The figure shows three views and two pictorial views of one solid part (mm, origin at its lowest corner). Answer the questions. Coordinates: 2 decimals unless noted, no trailing zeros. Loops run counter-clockwise (first coordinate to the right, second up) from the corner with the lowest first, then second, coordinate; pieces in that order, holes last. Notation, with made-up numbers: (30.5, -9) -> (43.5, -9) arc R8 cw to (43.5, 6) -> close; hole circle Ø10 at (89.25, -9). An arc over 180 degrees is marked (long way). Answer in a Markdown table with one row per item.
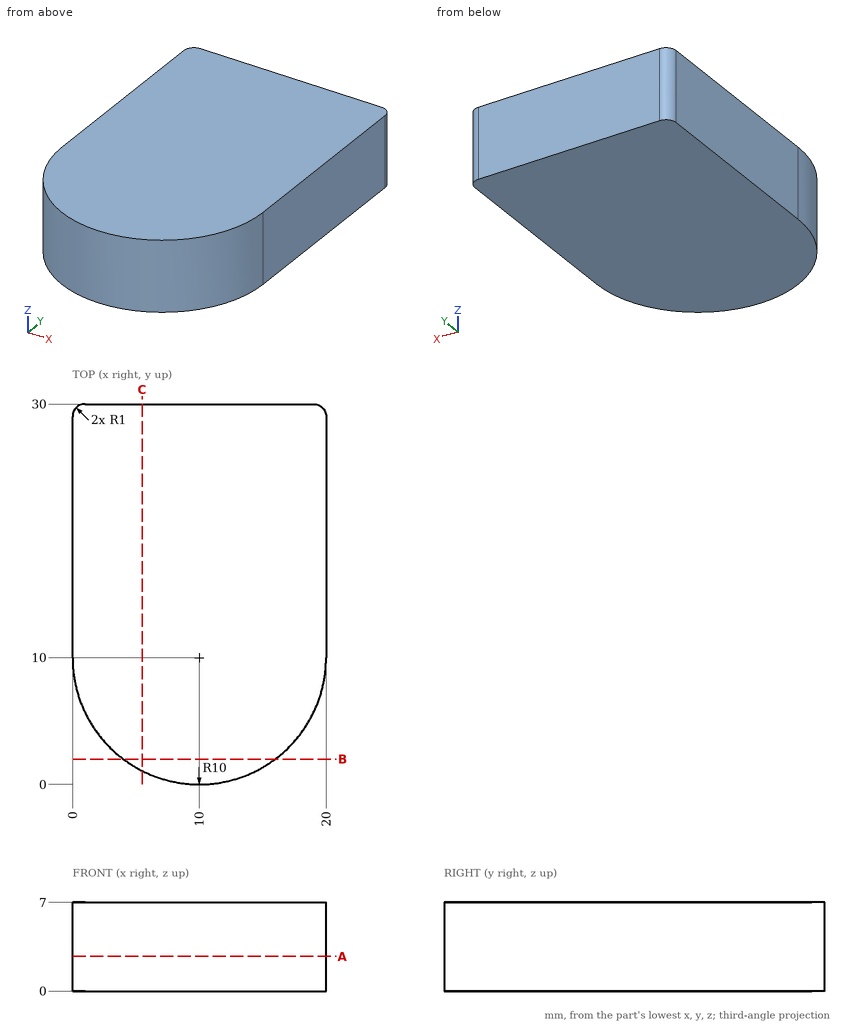
Item 1: A cutting plane is placed at B-B, the plane y = 2. Determine the outline of the cut face in (x, z), plus the area to 3 significant figures.
Findings below:
| item | result |
|---|---|
| outline | (4, 0) -> (16, 0) -> (16, 7) -> (4, 7) -> close |
| area | 84.0 mm2 |
Item 2: A cutting plane is placed at A-A, the plane z = 2.75. Determine the outline of the cut face in (x, y), plus the area to 3 significant figures.
Findings below:
| item | result |
|---|---|
| outline | (0, 10) arc R10 ccw to (20, 10) -> (20, 29) arc R1 ccw to (19, 30) -> (1, 30) arc R1 ccw to (0, 29) -> close |
| area | 557 mm2 |
Item 3: Flat-ended cylindrical pins translate along their axes: pin 1 Ø1.5 at (x, y) = (10.5, 3.5) entering from -Z; pin 2 Ø1 at (x, z) = (5, 3.5) entering from -Y. Find the tip coordinate at first contact, or state that the pin passes through.
Findings below:
| item | result |
|---|---|
| pin 1 | stops at z = 0 |
| pin 2 | stops at y = 1.07 |
Item 4: A cutting plane is placed at C-C, the plane x = 5.5. Determine the outline of the cut face in (y, z), plus the area to 3 significant figures.
Findings below:
| item | result |
|---|---|
| outline | (1.07, 0) -> (30, 0) -> (30, 7) -> (1.07, 7) -> close |
| area | 203 mm2 |
Item 5: Find the intervals of material crossed by probe 1 along Y at (x, z) = (10.25, 4); probe 2 along X at (y, z) = (9.75, 5.5); probe 3 along Y at (x, z) = (13, 1.5), in increasing order.
Findings below:
| item | result |
|---|---|
| probe 1 | y = 0 to 30 |
| probe 2 | x = 0 to 20 |
| probe 3 | y = 0.46 to 30 |
